```python
from build123d import *

# Parameters (mm, degrees)
F0_W     = 152.4
F0_H     = 203.2
F1_DEPTH = 12.7
F2_W     = 15.24
F2_H     = 203.2
F3_DEPTH = 5.08
F5_DEPTH = 203.2
F7_DEPTH = 5.08
F9_DEPTH = 5.08


with BuildPart() as f1:
    # F0 (on Front) → F1 (new body, symmetric)
    with BuildSketch(Plane.XZ):
        with Locations((-30.4995095253, 70.9851061165)):
            Rectangle(F0_W, F0_H)
    extrude(amount=F1_DEPTH, both=True)

    # F2 (on face) → F3 (cut)
    with BuildSketch(Plane.YZ.offset(45.7004904747)):
        with Locations((0, 70.9851061165)):
            Rectangle(F2_W, F2_H)
    extrude(amount=-F3_DEPTH, mode=Mode.SUBTRACT)

    # F4 (on face) → F5 (join)
    with BuildSketch(Plane.XY.offset(172.5851061165)):
        with BuildLine():
            Line((-106.6995095253, -12.7), (-106.6995095253, 12.7))
            ThreePointArc((-106.6995095253, 12.7), (-110.5322322417, 0), (-106.6995095253, -12.7))
        make_face()
    extrude(amount=-F5_DEPTH)

    # F6 (on face) → F7 (cut)
    with BuildSketch(Plane.XY.offset(172.5851061165)):
        with BuildLine():
            Line((40.6204904747, 7.62), (-103.746953477, 7.62))
            ThreePointArc((-103.746953477, 7.62), (-105.4522322417, 0), (-103.746953477, -7.62))
            Line((-103.746953477, -7.62), (40.6204904747, -7.62))
            Line((40.6204904747, -7.62), (40.6204904747, 7.62))
        make_face()
    extrude(amount=-F7_DEPTH, mode=Mode.SUBTRACT)

    # F8 (on face) → F9 (cut)
    with BuildSketch(Plane(origin=(0, 0, -30.6148938835), x_dir=(1, 0, 0), z_dir=(0, 0, -1))):
        with BuildLine():
            ThreePointArc((-103.746953477, 7.62), (-105.4522322417, 0), (-103.746953477, -7.62))
            Line((-103.746953477, -7.62), (40.6204904747, -7.62))
            Line((40.6204904747, -7.62), (40.6204904747, 7.62))
            Line((40.6204904747, 7.62), (-103.746953477, 7.62))
        make_face()
    extrude(amount=-F9_DEPTH, mode=Mode.SUBTRACT)


solid = f1.part
```
The listing builds one solid part. Answer for the finished solid, in the listing's coordinates (mm). A direction names the side the tool comes from. Round coordinates to 2 decimals unless told otherwise and drop trailing zeros. Loops run counter-clockwise (first coordinate to the right, second up) from the corner with the lowest first, then second, coordinate; pieces in that order, holes last.
1) For faces 1 (the face through (40.62, 0, 72)), 2 (the face through (-110.53, 0.19, 72.41)), 3 (the face through (43, -7.62, 71)), 4 (the face through (-33, 0, 167.505)), 5 (the face through (-33, 0, -25.535)), determine the directions among +Z, -Z, +X, -X, +Y, -Y from which every point of the face is accessible in a straight line to the end or side of a thin tool.
Outcome:
face 1: +Z, -Z, +X
face 2: +Z, -Z, -X
face 3: +X
face 4: +Z, +X
face 5: -Z, +X
2) A cutting plane is placed at B-B on y = -1.25. Determine the outline of the cut face in (x, z).
Outcome:
outline: (-110.5, -30.61) - (-105.41, -30.61) - (-105.41, -25.53) - (40.62, -25.53) - (40.62, 167.51) - (-105.41, 167.51) - (-105.41, 172.59) - (-110.5, 172.59) - close
3) Consider line 1 (Z direction, x = 28.5, y = 5.25); line 2 (X direction, y = -1, z = 134); line 3 (X direction, y = 8.75, z = 49). Determine where each line is inside the solid, lowest interval first.
Outcome:
line 1: z = -25.53 to 167.51
line 2: x = -110.51 to 40.62
line 3: x = -108.8 to 45.7
4) A cutting plane is placed at C-C on x = -39.5. Determine the outline of the cut face in (y, z), plus the area to 3 significant figures.
Outcome:
outline: (-12.7, -30.61) - (-7.62, -30.61) - (-7.62, -25.53) - (7.62, -25.53) - (7.62, -30.61) - (12.7, -30.61) - (12.7, 172.59) - (7.62, 172.59) - (7.62, 167.51) - (-7.62, 167.51) - (-7.62, 172.59) - (-12.7, 172.59) - close
area: 5,010 mm2
5) Given P1, Ø2, axis at y = -4, z = 56, coming from the -X side; P2, Ø8, axis at y = 1.5, z = 24.5, coming from the +X side; P3, Ø1.5, axis at x = -56, y = -7, coming from the +Z side; P4, Ø6, axis at y = 5.5, z = 70, coming from the -X side, each flat-ended and moving along its own axis, determine where each tip first touches the part or whether it passes through.
Outcome:
P1: stops at x = -110.34
P2: stops at x = 40.62
P3: stops at z = 172.59
P4: stops at x = -110.4
6) For a pull along Y with two mould halves and no side action, classify faces 6 (the face through (43, 7.62, 71)), 7 (the face through (-105.45, 0.11, 170.08)), 8 (the face through (-32, 12.7, 72)), 9 (the face through (-34, 9, -30.615)) as released by +Y, released by -Y, zero draft, split by the parting line, or undercut.
Outcome:
face 6: undercut
face 7: undercut
face 8: released by +Y
face 9: zero draft
7) A cutting plane is placed at A-A on z = 129. Determine the outline of the cut face in (x, y), plus the area to 3 significant figures.
Outcome:
outline: (-106.7, -12.7) - (45.7, -12.7) - (45.7, -7.62) - (40.62, -7.62) - (40.62, 7.62) - (45.7, 7.62) - (45.7, 12.7) - (-106.7, 12.7) arc R22.96 ccw to start
area: 3,860 mm2
